Build history of the part. All positions in model axes, mm. A direction names the side the tool comes from. Give positions to 0.01 mm unless a question says otherwise; leave off trailing zeros. Loops run counter-clockwise (first coordinate to the right, second up) from the corner with the lowest first, then second, coordinate; pieces in that order, holes last. Notation, with made-up numbers: M 32.5,-10 L 61.5,-10 A11 cw 61.5,11 Z; hole C 83,17 d11. An arc over 180 degrees is marked long. Answer in a Markdown table with one row per item. Add a question column.
```python
from build123d import *

# Parameters (mm, degrees)
F1_DEPTH = 63.5
F2_DEPTH = 25.4
F3_DEPTH = 7.9375
F0_W     = 25.5843524362
F0_H     = 19.05
F4_DEPTH = 25.4
F6_R     = 6.35


with BuildPart() as f1:
    # F0 (on Front) → F1 (new body, symmetric)
    with BuildSketch(Plane.XZ):
        Polygon((41.275, -9.525), (41.275, 9.525), (-22.225, 9.525), (-41.275, 9.525), (-41.275, -9.525), align=None)
    extrude(amount=F1_DEPTH, both=True)

    # F0 (on Front) → F2 (join, symmetric)
    with BuildSketch(Plane.XZ):
        with BuildLine():
            Line((-41.275, 9.525), (-22.225, 9.525))
            Line((-22.225, 9.525), (-22.225, 27.0002))
            ThreePointArc((-22.225, 27.0002), (-31.815718959, 51.0403711544), (-55.3204805517, 61.8772480917))
            add(Edge.make_bspline(
                [(-55.3204805517, 61.8772480917), (-55.929805309, 61.8954627703), (-56.5396707352, 61.9114442844), (-57.15, 61.9252)],
                knots=[110.1454497183, 110.1454497183, 110.1454497183, 110.1454497183, 111.5045361635, 111.5045361635, 111.5045361635, 111.5045361635], degree=3))
            Line((-57.15, 61.9252), (-60.325, 61.9252))
            Line((-60.325, 61.9252), (-60.325, 42.8752))
            Line((-60.325, 42.8752), (-57.15, 42.8752))
            ThreePointArc((-57.15, 42.8752), (-45.9246798487, 38.2255201513), (-41.275, 27.0002))
            Line((-41.275, 27.0002), (-41.275, 9.525))
        make_face()
    extrude(amount=F2_DEPTH, both=True)

    # F0 (on Front) → F3 (join, symmetric)
    with BuildSketch(Plane.XZ):
        with BuildLine():
            Line((-22.225, 9.525), (41.275, 9.525))
            add(Edge.make_bspline(
                [(41.275, 9.525), (39.8922745283, 44.2572563943), (-5.9385227977, 60.4010623985), (-55.3204805517, 61.8772480917)],
                knots=[0, 0, 0, 0, 110.1454497183, 110.1454497183, 110.1454497183, 110.1454497183], degree=3))
            ThreePointArc((-55.3204805517, 61.8772480917), (-31.815718959, 51.0403711544), (-22.225, 27.0002))
            Line((-22.225, 27.0002), (-22.225, 9.525))
        make_face()
    extrude(amount=F3_DEPTH, both=True)

    # F0 (on Front) → F4 (join, symmetric)
    with BuildSketch(Plane.XZ):
        with Locations((-73.1171762181, 52.4002)):
            Rectangle(F0_W, F0_H)
    extrude(amount=F4_DEPTH, both=True)

    # F0 (on Front) → F5 (revolve)
    with BuildSketch(Plane.XZ):
        Polygon((-85.9093524362, 42.8752), (-85.9093524362, 61.9252), (-85.9093524362, 66.675), (-111.125, 66.675), (-111.125, 38.1), (-85.9093524362, 38.1), align=None)
    revolve(axis=Axis((-85.9093524362, 0, 52.3875), (0, 0, -1)))

    # F6
    f6_edges = [f1.edges().sort_by_distance(p)[0] for p in [
        (41.275, 63.5, 0),
        (-41.275, 63.5, 0),
        (-41.275, -63.5, 0),
        (41.275, -63.5, 0),
    ]]
    fillet(f6_edges, radius=F6_R)


solid = f1.part
```
(1) Tool access for faces 4 (the flat face through (3, 7.938, 30)), 5 (the flat face through (-41.275, -1, 5)), 6 (the flat face through (0, -63.5, 0)), 7 (the flat face through (-22.225, -17, 18)): list every direction of +Z, -Z, +X, -X, +Y, -Y with a clear straight run to the whole face (end or side of a thin tool).
(2) Slice it at A-A, the plane z = 2. Give the cut face in (x, y) (3 decimals).
(3) Slice it at B-B, the plane y = 39. Give the cut face in (x, z) (3 decimals).
(4) Pin check, flat tips, straight feed: pin 1 (1.5 mm diameter, centred on x = -21, y = -40, fed in from +Z) (3 decimals); pin 2 (14 mm diameter, centred on y = 15, z = 22.5, fed in from +X) (3 decimals); pin 3 (8 mm diameter, centred on x = -27.5, z = 10, fed in from -Y); pin 4 (10 mm diameter, centred on y = 16.5, z = 47, fed in from -X). Stop position of each tip, or through.
(5) Wall check: line 1 (Z direction, x = 25, y = -27) (3 decimals); line 2 (X direction, y = -11, z = 8.5) (3 decimals); line 3 (Y direction, x = 17, z = 24). Give the ranges that are in metal, low to high.
(6) Pull direction X, two halves, no side cores. Call faces 1 (the cylindrical face through (-46, -0.4, 38.3)), 2 (the flat face through (-60, 0, 61.925)), 3 (the cylindrical face through (-31.56, -16.79, 50.77)): +X half, -X half, draft (parallel to the pull), parting line (faces both ways), or undercut.
Solution:
| question | item | result |
|---|---|---|
| 1 | face 4 | +Z, +X, +Y |
| 1 | face 5 | -Z, -X, +Y, -Y |
| 1 | face 6 | +Z, -Z, +X, -X, -Y |
| 1 | face 7 | +Z, +X, -Y |
| 2 | outline | M -41.275,-57.15 A6.35 ccw -34.925,-63.5 L 34.925,-63.5 A6.35 ccw 41.275,-57.15 L 41.275,57.15 A6.35 ccw 34.925,63.5 L -34.925,63.5 A6.35 ccw -41.275,57.15 Z |
| 3 | outline | M -41.275,-9.525 L 41.275,-9.525 L 41.275,9.525 L -41.275,9.525 Z |
| 4 | pin 1 | z = 9.525 |
| 4 | pin 2 | x = -22.225 |
| 4 | pin 3 | y = -63.5 |
| 4 | pin 4 | x = -108.35 |
| 5 | line 1 | -9.525 to 9.525 |
| 5 | line 2 | -41.275 to 41.275 |
| 5 | line 3 | -7.94 to 7.94 |
| 6 | face 1 | undercut |
| 6 | face 2 | draft |
| 6 | face 3 | +X half |
